The model under review builds one solid part; all positions refer to its coordinate system, in mm. A direction names the side the tool comes from. Give positions to 0.01 mm unless a question says otherwise; leave off trailing zeros. Loops run counter-clockwise (first coordinate to the right, second up) from the corner with the lowest first, then second, coordinate; pieces in that order, holes last. Notation, with made-up numbers: M 17,47.5 L 68,47.5 A15 cw 68,68.5 Z; hole C 75.5,50 d2. An arc over 180 degrees is marked long. Return JSON: item names as keys, results as strings.
Autodesk Inventor part; units mm, degrees
ref_plane "YZ Plane" through (0, 0, 0) normal (1, 0, 0) x (0, 1, 0)
ref_plane "XZ Plane" through (0, 0, 0) normal (0, 1, 0) x (-1, 0, 0)
ref_plane "XY Plane" through (0, 0, 0) normal (0, 0, 1) x (1, 0, 0)
sketch "Sketch1" plane through (0, 0, 0) normal (0, 0, 1) x (1, 0, 0)
  circle A0 centre (0, 0) radius 40
  dimension "d0" = 80
extrude "Extrusion1" add sketch "Sketch1" along normal blind 22.5
sketch "Sketch2" plane through (0, 0, 22.5) normal (0, 0, 1) x (1, 0, 0)
  point P0 (0, 0)
  point P1 (0, 35)
  dimension "d3" = 35
hole "Hole1" at (0, 35, 22.5) direction (0, 0, -1) diameter 4.3 end through all counterbore diameter 10.59 counterbore depth 5
chamfer "Chamfer1" distance 2 distance2 3 2 edges at (-27.6179, -28.9353, 22.5) (28.9353, 27.6179, 22.5) measured on face at (-2.7418, -16.4668, 22.5)
pattern_circular "Circular Pattern1" count 6 over 360 about axis through (0, 0, 0) along (0, 0, 1) of "Hole1"
sketch "Sketch3" plane through (0, 0, 0) normal (0, 0, -1) x (-1, 0, 0)
  circle A0 centre (0, 0) radius 29.1
  dimension "d17" = 58.2
extrude "Extrusion2" cut sketch "Sketch3" against normal through all
ref_plane "Work Plane1" through (0, 0, 10.5) normal (0, 0, -1) x (-1, 0, 0)
sketch "Sketch4" plane through (0, 0, 10.5) normal (0, 0, -1) x (-1, 0, 0)
  circle A0 centre (0, 0) radius 29.5
  circle A1 centre (0, 0) radius 26.5
  dimension "d21" = 53
  dimension "d22" = 59
extrude "Extrusion3" add sketch "Sketch4" against normal blind 3
sketch "Sketch5" plane through (0, 0, 22.5) normal (0, 0, 1) x (1, 0, 0)
  arc A0 (33.6722, 21.5913) -> (1.8625, 39.9566) centre (0, 0) ccw
  line L0 (0, 0) -> (40, 0) construction
  line L1 (21.4926, 23.7527) -> (24.6091, 28.2845)
  line L2 (24.6091, 28.2845) -> (17.6054, 33.101)
  line L3 (17.6054, 33.101) -> (14.4889, 28.5691)
  line L4 (14.4889, 28.5691) -> (21.4926, 23.7527)
  line L5 (21.4926, 23.7527) -> (17.6054, 33.101) construction
  line L6 (24.6091, 28.2845) -> (14.4889, 28.5691) construction
  line L7 (17.002, 26.8409) -> (20.1185, 31.3727)
  line L8 (22.1372, 29.9845) -> (19.0207, 25.4526)
  line L9 (14.8714, 29.1253) -> (17.223, 32.5448)
  line L10 (17.223, 32.5448) -> (19.736, 30.8165)
  line L11 (19.736, 30.8165) -> (17.3845, 27.3971)
  line L12 (17.3845, 27.3971) -> (14.8714, 29.1253)
  line L13 (19.549, 28.4268) -> (16.0472, 30.8351)
  line L14 (17.3845, 27.3971) -> (17.223, 32.5448)
  line L15 (14.8714, 29.1253) -> (19.736, 30.8165)
  line L16 (0, 0) -> (17.3037, 29.9709)
  line L17 (0, 0) -> (19.549, 28.4268)
  dimension "d26" = 8.5
  dimension "d27" = 5.5
  dimension "d29" = 34.5
  dimension "d30" = 3.05
  dimension "d36" = 3
  dimension "d41" = 4.15
  dimension "d42" = 60
extrude "Extrusion4" cut sketch "Sketch5" against normal blind 1.75 contours L4 L17 L13 L7 L2 L8 | L4 L7 L13 L17 | L15 L14 L10 | L7 L13 L15 | L14 L13 L7 | L12 L16 L14 | L14 L13 L3 | L15 L3 L13 | L16 L12 L15
extrude "Extrusion7" cut sketch "Sketch5" against normal through all contours L4 L8 L2 L1
properties part number "Ring Cover Top"
1) Consider section B-B on y = 0. Write out the cut boundary in (x, z), then the cut area to 3 significant figures.
From the geometry:
{"outline": "M -40,0 L -29.1,0 L -29.1,10.5 L -26.5,10.5 L -26.5,13.5 L -29.1,13.5 L -29.1,22.5 L -38,22.5 L -40,19.5 Z; M 26.5,10.5 L 29.1,10.5 L 29.1,0 L 40,0 L 40,19.5 L 38,22.5 L 29.1,22.5 L 29.1,13.5 L 26.5,13.5 Z", "area": "500 mm²"}
2) The part is to be moulded in two halves that separate along Y. For faces 4 (the face through (-8.67, 39.05, 9.61)), 5 (the face through (23.393, 29.121, 11.408)), 6 (the face through (-27, -12, 0)), say which applies: released by +Y, released by -Y, zero draft, split by the parting line, or undercut.
From the geometry:
{"face 4": "split by the parting line", "face 5": "undercut", "face 6": "zero draft"}
3) Wall thickness on L1, parallel to Y at x = 23.5, z = 2; L2, parallel to Y at x = -29.5, z = 2.25; L3, parallel to X at y = -15, z = 21.5: over which ranges is each line inside the solid? List them lowest first. Write a range as from..to.
From the geometry:
{"L1": "-32.37..-17.16, 17.16..26.67, 29.05..32.37", "L2": "-27.01..-19.49, -15.51..15.51, 19.49..27.01", "L3": "-35.64..-34.98, -25.64..-24.94, 24.94..25.64, 34.98..35.64"}
4) Consider section C-C on z = 8.5. Count the separate pieces of the cut face and the enclosed holes in it, then the cut area to 3 significant figures.
From the geometry:
{"separate pieces": "1", "enclosed holes": "8", "area": "2,260 mm²"}
5) Consider section A-A on x = 0. Write out the cut boundary in (y, z) (3 decimals).
From the geometry:
{"outline": "M -40,0 L -37.15,0 L -37.15,17.5 L -40,17.5 Z; M -32.85,0 L -29.1,0 L -29.1,10.5 L -26.5,10.5 L -26.5,13.5 L -29.1,13.5 L -29.1,22.5 L -29.705,22.5 L -29.705,17.5 L -32.85,17.5 Z; M 26.5,10.5 L 29.1,10.5 L 29.1,0 L 32.85,0 L 32.85,17.5 L 29.705,17.5 L 29.705,22.5 L 29.1,22.5 L 29.1,13.5 L 26.5,13.5 Z; M 37.15,0 L 40,0 L 40,17.5 L 37.15,17.5 Z"}
6) Insertion check: pin 1 (3 mm diameter, centred on x = 1, y = 37, fed in from +Z); pin 2 (4 mm diameter, centred on y = 12, z = 8, fed in from -X); pin 3 (5 mm diameter, centred on x = 24.5, z = 3.5, fed in from +Y). Each pin has a flat end and moves straight along its axis. Give the tip position at first contact, or say it passes through.
From the geometry:
{"pin 1": "z = 17.5", "pin 2": "x = -38.73", "pin 3": "y = 33.41"}
7) Tool access review of faces 1 (the face through (-31, -15, 17.5)), 2 (the face through (-0.65, 32.95, 8.63)), 3 (the face through (26, 7, 10.5)): name each direction out of +Z, -Z, +X, -X, +Y, -Y from which nothing blocks a thin tool from reaching the whole face with its end or side.
From the geometry:
{"face 1": "+Z", "face 2": "+Z, -Z", "face 3": "-Z"}
